Geometry check sheet. Reference: the model listing, model coordinates, mm. Face numbers are marked on the shaded views. A direction names the side the tool comes from. Coordinates: 2 decimals unless noted, no trailing zeros. Loops run counter-clockwise (first coordinate to the right, second up) from the corner with the lowest first, then second, coordinate; pieces in that order, holes last. Notation, with made-up numbers: (49, 20.5) - (74, 20.5) arc R27 cw to (74, 41.5) - close; hole circle Ø10 at (30, -24.5). An arc over 180 degrees is marked (long way). Write each question's results on one line, items separated by ' | '. Start each with the question number.
(1) Sectioned sample at B-B (x = 18.75). Enter the section's corners in (y, z), plus the area to 3 significant figures.
(2) Go/stop test with flat-tipped pins: pin 1 Ø1.5 at (x, y) = (3.5, -8) entering from +Z; pin 2 Ø4 at (x, z) = (14, 0) entering from -Y; pin 3 Ø2 at (x, z) = (4, 2) entering from -Y. Record where each tip stops, or that it passes through.
(3) Access from +Z, -Z, +X, -X, +Y, -Y to the whole of each face (thin tool, end or side, straight path). Record for the marked faces 1 and 2.
(4) Sectioned sample at A-A (z = 0). Enter the section's corners in (x, y), plus the area to 4 significant figures.
(5) Material ranges on probe 1 along X at (y, z) = (-10.75, 2.25); probe 2 along Y at (x, z) = (1.05, 4.25); probe 3 along Z at (x, y) = (3.5, 6), recorded low to high.
(6) Mould release check, pull along Z, two halves, no side actions. Record for the marked faces 3, 4 and 5: pulls with the +Z half, pulls with the -Z half, needs draft (parallel to the pull), parting line crosses it, or undercut.
from build123d import *

# Parameters (mm, degrees)
SKIZZE2_R                            = 10
AUFSATZ_LINEAR_AUSTRAGEN1_DEPTH      = 25
SKIZZE3_R                            = 12
AUFSATZ_LINEAR_AUSTRAGEN2_DEPTH      = 2
SCHNITT_LINEAR_AUSTRAGEN1_DEPTH      = 15
FASE1_SIZE                           = 1
FASE2_SIZE                           = 1
F_3_1_3_1_DURCHMESSER_BOHRUNG1_D     = 3.1
F_3_1_3_1_DURCHMESSER_BOHRUNG1_DEPTH = 7
F_3_1_3_1_DURCHMESSER_BOHRUNG1_TIP   = 0.931333959
FASE3_SIZE                           = 1


with BuildPart() as part:
    # Skizze2 → Aufsatz-Linear austragen1 (new body)
    with BuildSketch(Plane(origin=(0, 0, 0), x_dir=(0, 0, -1), z_dir=(1, 0, 0))):
        Circle(SKIZZE2_R)
    extrude(amount=AUFSATZ_LINEAR_AUSTRAGEN1_DEPTH)

    # Skizze3 → Aufsatz-Linear austragen2 (add)
    with BuildSketch(Plane.ZY):
        Circle(SKIZZE3_R)
    extrude(amount=AUFSATZ_LINEAR_AUSTRAGEN2_DEPTH)

    # Skizze4 → Schnitt-Linear austragen1 (cut)
    with BuildSketch(Plane(origin=(25, 0, 0), x_dir=(0, 0, -1), z_dir=(1, 0, 0))):
        with BuildLine():
            Line((-1.774823935, 1.9), (1.774823935, 1.9))
            ThreePointArc((1.774823935, 1.9), (0, -2.6), (-1.774823935, 1.9))
        make_face()
    extrude(amount=-SCHNITT_LINEAR_AUSTRAGEN1_DEPTH, mode=Mode.SUBTRACT)

    # Fase1
    fase1_edges = [part.edges().sort_by_distance(p)[0] for p in [
        (25, -2.6, 0),
        (25, 1.9, 0),
    ]]
    chamfer(fase1_edges, length=FASE1_SIZE)

    # Fase2
    fase2_edges = [part.edges().sort_by_distance(p)[0] for p in [
        (25, 0, 10),
    ]]
    chamfer(fase2_edges, length=FASE2_SIZE)

    # Ø3.1 (3.1) Durchmesser Bohrung1
    with Locations(Plane.ZY.offset(2)):
        with Locations((4.25, 0), (-4.25, 0)):
            Hole(F_3_1_3_1_DURCHMESSER_BOHRUNG1_D / 2, depth=F_3_1_3_1_DURCHMESSER_BOHRUNG1_DEPTH)
            with Locations((0, 0, -(F_3_1_3_1_DURCHMESSER_BOHRUNG1_DEPTH + F_3_1_3_1_DURCHMESSER_BOHRUNG1_TIP / 2))):  # 118° drill point
                Cone(0, F_3_1_3_1_DURCHMESSER_BOHRUNG1_D / 2, F_3_1_3_1_DURCHMESSER_BOHRUNG1_TIP, mode=Mode.SUBTRACT)

    # Fase3
    fase3_edges = [part.edges().sort_by_distance(p)[0] for p in [
        (-2, 0, 5.8),
        (-2, 0, -2.7),
    ]]
    chamfer(fase3_edges, length=FASE3_SIZE)


solid = part.part
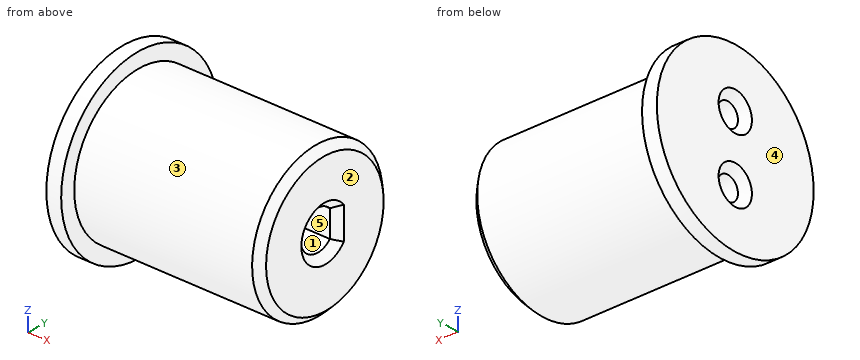
Outcome:
1) outline: circle Ø20 at (0, 0); hole (1.9, -1.77) - (1.9, 1.77) arc R2.6 ccw (long way) to start | area: 295 mm2
2) pin 1: stops at z = 6.89 | pin 2: stops at y = -10 | pin 3: stops at y = -9.95
3) face 1: +X | face 2: +Z, -Z, +X, +Y, -Y
4) outline: (-2, -12) - (0, -12) - (0, -10) - (24, -10) - (25, -9) - (25, -3.6) - (24, -2.6) - (10, -2.6) - (10, 1.9) - (24, 1.9) - (25, 2.9) - (25, 9) - (24, 10) - (0, 10) - (0, 12) - (-2, 12) - close | area: 478.5 mm2
5) probe 1: x = -2 to 0 | probe 2: y = -9.05 to -1.55, 1.55 to 9.05 | probe 3: z = -8 to 8
6) face 3: parting line crosses it | face 4: needs draft | face 5: undercut
